```python
from build123d import *

# Parameters (mm, degrees)
F0_R      = 12.5
F1_DEPTH  = 15
F2_R      = 10.75
F3_DEPTH  = 5
F4_R      = 7
F5_DEPTH  = 5
F6_R      = 0.7
F8_DEPTH  = 2
F9_R      = 0.75
F10_DEPTH = 15


with BuildPart() as f1:
    # F0 (on Front) → F1 (new body)
    with BuildSketch(Plane.XZ):
        Circle(F0_R)
        Polygon((-3.897114317, -2.25), (0, 4.5), (3.897114317, -2.25), align=None, mode=Mode.SUBTRACT)
    extrude(amount=F1_DEPTH)

    # F2 (on face) → F3 (cut)
    with BuildSketch(Plane(origin=(0, 0, 0), x_dir=(-1, 0, 0), z_dir=(0, 1, 0))):
        Circle(F2_R)
        Polygon((-3.897114317, -2.25), (0, 4.5), (3.897114317, -2.25), align=None, mode=Mode.SUBTRACT)
    extrude(amount=-F3_DEPTH, mode=Mode.SUBTRACT)

    # F4 (on face) → F5 (cut)
    with BuildSketch(Plane(origin=(0, -5, 0), x_dir=(-1, 0, 0), z_dir=(0, 1, 0))):
        Circle(F4_R)
    extrude(amount=-F5_DEPTH, mode=Mode.SUBTRACT)

    # F6
    f6_edges = [f1.edges().sort_by_distance(p)[0] for p in [
        (0, -12.5, 4.5),
        (-3.897114, -12.5, -2.25),
        (3.897114, -12.5, -2.25),
    ]]
    fillet(f6_edges, radius=F6_R)

    # F7 (on face) → F8 (join)
    with BuildSketch(Plane(origin=(0, 0, 0), x_dir=(-1, 0, 0), z_dir=(0, 1, 0))):
        with BuildLine():
            ThreePointArc((-10.7057848837, -0.973996932), (-10.0451118038, -0.6736153434), (-9.775, 0))
            ThreePointArc((-9.775, 0), (-10.0451118038, 0.6736153434), (-10.7057848837, 0.973996932))
            ThreePointArc((-10.7057848837, 0.973996932), (-10.75, 0), (-10.7057848837, -0.973996932))
        make_face()
        with BuildLine():
            ThreePointArc((10.75, 0), (10.738940532, 0.4875), (10.7057848837, 0.973996932))
            ThreePointArc((10.7057848837, 0.973996932), (9.775, 0), (10.7057848837, -0.973996932))
            ThreePointArc((10.7057848837, -0.973996932), (10.738940532, -0.4875), (10.75, 0))
        make_face()
    extrude(amount=-F8_DEPTH)

    # F9 (on Front) → F10 (join)
    with BuildSketch(Plane.XZ):
        with Locations((-10.3421816602, 6.477789022)):
            Circle(F9_R)
        with BuildLine():
            ThreePointArc((0.3111609767, -12.1954865593), (0.2288544945, -11.8538941615), (0, -11.5872758133))
            Line((0, -11.5872758133), (0, -12.8036973054))
            ThreePointArc((0, -12.8036973054), (0.2288544945, -12.5370789572), (0.3111609767, -12.1954865593))
        make_face()
        with BuildLine():
            Line((0, -12.8036973054), (0, -11.5872758133))
            ThreePointArc((0, -11.5872758133), (-1.1888390233, -12.1954865593), (0, -12.8036973054))
        make_face()
        with Locations((-12.0864133121, -1.6855519443)):
            Circle(F9_R)
        with Locations((-8.1752778497, -9.0602044231)):
            Circle(F9_R)
        with Locations((7.5029374592, -9.6243649967)):
            Circle(F9_R)
        with Locations((11.9340061187, -2.5498960893)):
            Circle(F9_R)
        with Locations((10.7810206836, 5.7176975373)):
            Circle(F9_R)
        with Locations((4.5834758529, 11.309916941)):
            Circle(F9_R)
        with Locations((-3.758728269, 11.6101005123)):
            Circle(F9_R)
    extrude(amount=F10_DEPTH)


solid = f1.part
```
Work out the finished part from the listing and answer in its coordinate system (mm). A direction names the side the tool comes from. Round coordinates to 2 decimals unless told otherwise and drop trailing zeros. Loops run counter-clockwise (first coordinate to the right, second up) from the corner with the lowest first, then second, coordinate; pieces in that order, holes last. Notation, with made-up numbers: (51, 77) -> (87, 77) arc R27 ccw to (87, 109) -> close; hole circle Ø10 at (-4.5, 19). An arc over 180 degrees is marked (long way). Write each question's results on one line, items separated by ' | '. Start each with the question number.
1. Find the intervals of material crossed by probe 1 along X at (y, z) = (-2.9, 0); probe 2 along Y at (x, z) = (1, -4.5); probe 3 along Y at (x, z) = (6.5, -4), in increasing order. Write a range as from..to.
2. Section B-B (y = -9.25) is taken. Determine the outline of the cut face in (x, z), plus the area to 3 significant figures.
3. For a pull along X with two mould halves and no side action, classify faces 4 (the face through (-11.067, -7.395, -5.811)), 5 (the face through (0, -15, -3)), 6 (the face through (-8.687, -7.395, -9.609)), 7 (the face through (8.41, -7.4, 9.25)) as +X half, -X half, draft (parallel to the pull), parting line (faces both ways), or undercut.
4. Section D-D (y = -13) is taken. Determine the outline of the cut face in (x, z).
5. Section A-A (x = 4.75) is taken. Determine the outline of the cut face in (y, z).
6. Section C-C (z = -8) is taken. Determine the outline of the cut face in (x, y), plus the area to 3 significant figures.
7. A tool of negligible diameter and unlimited length cuts with its end or side. For faces 1 (the face through (-6.466, -7.465, -2.681)), 2 (the face through (10, -2, 0)), 3 (the face through (3.286, -12.535, -1.909)), from which of +Z, -Z, +X, -X, +Y, -Y can it reach the whole face along a straight path? Write none if from no direction.
8. Given pin 1 Ø3 at (x, y) = (2, -5) entering from -Z; pin 2 Ø1 at (x, z) = (-2.5, -4) entering from +Y; pin 3 Ø5 at (x, z) = (1.5, 6.5) entering from +Y, each flat-ended and moving along its own axis, determine where each tip first touches the part or whether it passes through.
Evaluation:
1) probe 1: x = -12.5..-10.75, 10.75..12.5 | probe 2: y = -15..-10 | probe 3: y = -15..-5
2) outline: (-12.46, -1.03) arc R0.75 ccw to (-12.26, -2.41) arc R12.5 ccw to (-8.88, -8.8) arc R0.75 ccw to (-7.84, -9.73) arc R12.5 ccw to (-1.15, -12.45) arc R0.75 ccw to (0.25, -12.5) arc R12.5 ccw to (7.12, -10.27) arc R0.75 ccw to (8.22, -9.41) arc R12.5 ccw to (12.06, -3.29) arc R0.75 ccw to (12.35, -1.93) arc R12.5 ccw to (11.35, 5.23) arc R0.75 ccw to (10.7, 6.46) arc R12.5 ccw to (5.33, 11.31) arc R0.75 ccw to (4.04, 11.83) arc R12.5 ccw to (-3.18, 12.09) arc R0.75 ccw to (-4.51, 11.66) arc R12.5 ccw to (-10.21, 7.22) arc R0.75 ccw to (-10.95, 6.03) arc R12.5 ccw to start; hole circle Ø14 at (0, 0) | area: 341 mm2
3) face 4: -X half | face 5: draft | face 6: undercut | face 7: +X half
4) outline: (-12.46, -1.03) arc R0.75 ccw to (-12.26, -2.41) arc R12.5 ccw to (-8.88, -8.8) arc R0.75 ccw to (-7.84, -9.73) arc R12.5 ccw to (-1.15, -12.45) arc R0.75 ccw to (0.25, -12.5) arc R12.5 ccw to (7.12, -10.27) arc R0.75 ccw to (8.22, -9.41) arc R12.5 ccw to (12.06, -3.29) arc R0.75 ccw to (12.35, -1.93) arc R12.5 ccw to (11.35, 5.23) arc R0.75 ccw to (10.7, 6.46) arc R12.5 ccw to (5.33, 11.31) arc R0.75 ccw to (4.04, 11.83) arc R12.5 ccw to (-3.18, 12.09) arc R0.75 ccw to (-4.51, 11.66) arc R12.5 ccw to (-10.21, 7.22) arc R0.75 ccw to (-10.95, 6.03) arc R12.5 ccw to start; hole (-3.29, -1.2) arc R0.7 ccw to (-2.68, -2.25) -> (2.68, -2.25) arc R0.7 ccw to (3.29, -1.2) -> (0.61, 3.45) arc R0.7 ccw to (-0.61, 3.45) -> close
5) outline: (-15, -11.56) -> (0, -11.56) -> (0, -9.64) -> (-5, -9.64) -> (-5, -5.14) -> (-10, -5.14) -> (-10, 5.14) -> (-5, 5.14) -> (-5, 9.64) -> (0, 9.64) -> (0, 12.04) -> (-15, 12.04) -> close
6) outline: (-9.6, -15) -> (9.6, -15) -> (9.6, 0) -> (7.18, 0) -> (7.18, -5) -> (-7.18, -5) -> (-7.18, 0) -> (-9.6, 0) -> close | area: 216 mm2
7) face 1: +Y | face 2: none | face 3: +Y, -Y
8) pin 1: stops at z = -12.49 | pin 2: stops at y = -10 | pin 3: stops at y = -5
